Can you work these out from the drawing? Everything is in mm from the part's minimum corner. Give positions to 0.01 mm unless a question says otherwise; leave off trailing zeros. Loops run counter-clockwise (first coordinate to the right, second up) from the corner with the lowest first, then second, coordinate; pieces in that order, holes last. Notation, with made-up numbers: (40, 29) - (71, 29) arc R20 ccw to (71, 65) - close; hole circle Ø4 at (-0.75, -22.5). An arc over 180 degrees is marked (long way). One line per item, written item: value. Start each with the question number.
Q1. If we mould it in two halves opening along Z, with no side actions, what happens to the marked faces 1, 2 and 3? For each: released by +Z, released by -Z, zero draft, split by the parting line, or undercut.
Q2. I want a section at A-A (x = 30). Please give me the cut outline in (y, z), then the cut area to 3 significant figures.
Q3. I want a section at B-B (y = 80). Please give me the cut outline in (x, z), then the cut area to 3 significant figures.
Q4. I'm going to push flat-ended pins straight in: P1, Ø4.5, axis at x = 10, y = 50, coming from the +Z side; P2, Ø3.5, axis at x = 10, y = 80, coming from the +Z side; P3, Ø4.5, axis at x = 10, z = 80, coming from the +Y side. Where does each tip first touch, or does it pass through?
Q5. If I drill on line 1 (Y direction, x = 30, z = 1.2); line 2 (Z direction, x = 26, y = 47), over which ranges is the centre line in solid material (lowest first)? Write a range as from..to.
Q6. I want a section at D-D (z = 62). Please give me the cut outline in (x, y).
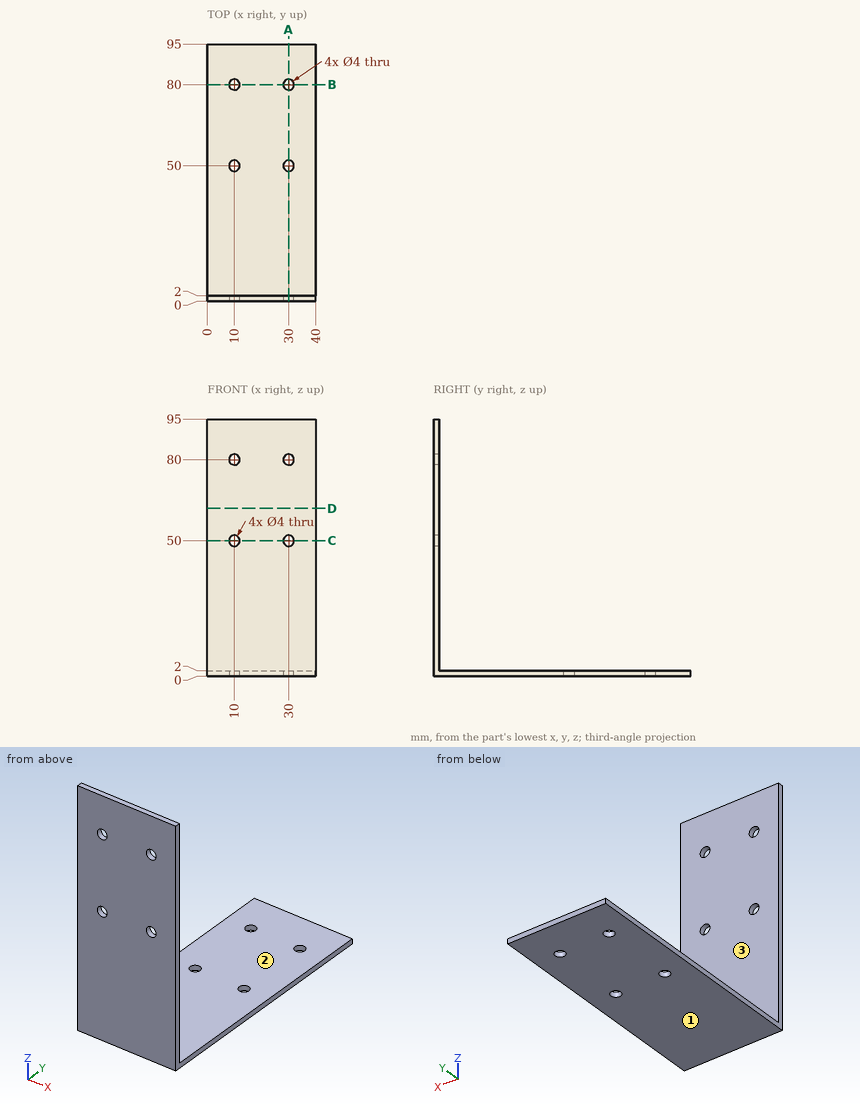
Worked answers:
1. face 1: released by -Z
1. face 2: released by +Z
1. face 3: zero draft
2. outline: (0, 0) - (48, 0) - (48, 2) - (2, 2) - (2, 48) - (0, 48) - close; (0, 52) - (2, 52) - (2, 78) - (0, 78) - close; (0, 82) - (2, 82) - (2, 95) - (0, 95) - close; (52, 0) - (78, 0) - (78, 2) - (52, 2) - close; (82, 0) - (95, 0) - (95, 2) - (82, 2) - close
2. area: 344 mm²
3. outline: (0, 0) - (8, 0) - (8, 2) - (0, 2) - close; (12, 0) - (28, 0) - (28, 2) - (12, 2) - close; (32, 0) - (40, 0) - (40, 2) - (32, 2) - close
3. area: 64.0 mm²
4. P1: stops at z = 2
4. P2: passes through
4. P3: stops at y = 2
5. line 1: y = 0..48, 52..78, 82..95
5. line 2: z = 0..2
6. outline: (0, 0) - (40, 0) - (40, 2) - (0, 2) - close
